```python
from build123d import *

# Parameters (mm, degrees)
SKETCH1_R           = 12
BOSS_EXTRUDE1_DEPTH = 26
FILLET1_R           = 1


with BuildPart() as part:
    # Sketch1 → Boss-Extrude1 (new body)
    with BuildSketch(Plane(origin=(0, 0, 0), x_dir=(1, 0, 0), z_dir=(0, 1, 0))):
        with Locations(Location((0, 0, 0), (0, 0, 90))):
            Circle(SKETCH1_R)
    extrude(amount=BOSS_EXTRUDE1_DEPTH)

    # Sketch2 → Revolve1 (revolve)
    with BuildSketch(Plane.XY, mode=Mode.PRIVATE) as revolve1_sk:
        with BuildLine():
            Line((0, 55.943780463), (0, 26))
            Line((0, 26), (12, 26))
            ThreePointArc((12, 26), (10.76980199, 31.292576415), (7.331439149, 35.5))
            ThreePointArc((7.331439149, 35.5), (11.357816692, 48.872983346), (0, 57))
            Line((0, 57), (0, 55.943780463))
        make_face()
    revolve(revolve1_sk.sketch.rotate(Axis((0, 55.943780463, 0), (0, -1, 0)), 270), axis=Axis((0, 55.943780463, 0), (0, -1, 0)))

    # Fillet1
    fillet1_edges = [part.edges().sort_by_distance(p)[0] for p in [
        (0, 35.5, 7.331439149),
    ]]
    fillet(fillet1_edges, radius=FILLET1_R)


solid = part.part
```
Input: part model. Units: mm. Frame: model coordinates. Give positions to 0.01 mm unless a question says otherwise; leave off trailing zeros. Order: outer loops, then holes, each group sorted by start corner. A loop starts at its lowest first (then second) coordinate and runs counter-clockwise, first axis right, second up. Notation, with made-up numbers: (78.25, -8.75) - (111.25, -8.75) arc R17 cw to (111.25, 24.25) - close; hole circle Ø7 at (62.5, -16). An arc over 180 degrees is marked (long way). Use a Markdown table: item, result.
(1) Line query: line 1 (Y direction, x = 3, z = -9.5); line 2 (Z direction, x = 0.5, y = 20.5); line 3 (Y direction, x = -2.5, z = -8.25). Output: solid intervals per line, ascending. Write a range as from..to.
Computed values:
| item | result |
|---|---|
| line 1 | y = 0..32.69, 38.31..51.69 |
| line 2 | z = -11.99..11.99 |
| line 3 | y = 0..34.35, 36.65..53.35 |
(2) Section query D-D (y = 52). Output: boundary loops of the cut face in (x, z).
Computed values:
| item | result |
|---|---|
| outline | circle Ø19.49 at (0, 0) |
(3) Section query C-C (y = 16). Output: boundary loops of the cut face in (x, z).
Computed values:
| item | result |
|---|---|
| outline | circle Ø24 at (0, 0) |
(4) Pin query (flat end, axial travel): pin 1 (1 mm diameter, centred on x = 6.5, y = 16.5, fed in from +Z); pin 2 (5 mm diameter, centred on x = -9.5, z = 3.5, fed in from +Y); pin 3 (4 mm diameter, centred on y = 38, z = 1, fed in from -X). Return the tip coordinate at first contact, or that it passes through.
Computed values:
| item | result |
|---|---|
| pin 1 | stops at z = 10.39 |
| pin 2 | stops at y = 54.27 |
| pin 3 | stops at x = -10.88 |
(5) Section query A-A (x = 10.25). Output: boundary loops of the cut face in (y, z).
Computed values:
| item | result |
|---|---|
| outline | (0, -6.24) - (26, -6.24) arc R6.24 ccw to (26, 6.24) - (0, 6.24) - close; circle Ø12.48 at (45, 0) |
(6) Section query B-B (z = -8.75). Output: boundary loops of the cut face in (x, y), then the cut area to 3 significant figures.
Computed values:
| item | result |
|---|---|
| outline | (-8.21, 0) - (8.21, 0) - (8.21, 26) arc R8.21 ccw to (-8.21, 26) - close; circle Ø16.42 at (0, 45) |
| area | 745 mm2 |
